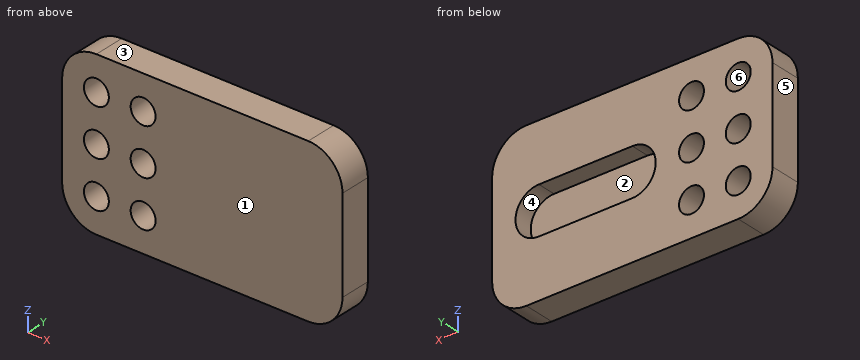
```python
from build123d import *

# Parameters (mm, degrees)
SKETCH1_W           = 180
SKETCH1_H           = 104
BOSS_EXTRUDE1_DEPTH = 20
FILLET1_R           = 22
SKETCH3_R           = 8
CUT_EXTRUDE1_DEPTH  = 20
CUT_EXTRUDE2_DEPTH  = 12


with BuildPart() as part:
    # Sketch1 → Boss-Extrude1 (new body)
    with BuildSketch(Plane(origin=(0, 0, 0), x_dir=(1, 0, 0), z_dir=(0, 1, 0))):
        Rectangle(SKETCH1_W, SKETCH1_H)
    extrude(amount=BOSS_EXTRUDE1_DEPTH)

    # Fillet1
    fillet1_edges = [part.edges().sort_by_distance(p)[0] for p in [
        (90, 10, 52),
        (-90, 10, 52),
        (-90, 10, -52),
        (90, 10, -52),
    ]]
    fillet(fillet1_edges, radius=FILLET1_R)

    # Sketch3 → Cut-Extrude1 (cut)
    with BuildSketch(Plane(origin=(0, 20, 0), x_dir=(1, 0, 0), z_dir=(0, 1, 0))):
        with Locations(Location((-68, 30, 0), (0, 0, 270))):
            Circle(SKETCH3_R)
        with Locations(Location((-68, 0, 0), (0, 0, 270))):
            Circle(SKETCH3_R)
        with Locations(Location((-68, -30, 0), (0, 0, 270))):
            Circle(SKETCH3_R)
        with Locations(Location((-38, -30, 0), (0, 0, 270))):
            Circle(SKETCH3_R)
        with Locations(Location((-38, 0, 0), (0, 0, 270))):
            Circle(SKETCH3_R)
        with Locations(Location((-38, 30, 0), (0, 0, 270))):
            Circle(SKETCH3_R)
    extrude(amount=-CUT_EXTRUDE1_DEPTH, mode=Mode.SUBTRACT)

    # Sketch4 → Cut-Extrude2 (cut)
    with BuildSketch(Plane(origin=(0, 20, 0), x_dir=(1, 0, 0), z_dir=(0, 1, 0))):
        with BuildLine():
            Line((0, 15), (60, 15))
            ThreePointArc((60, 15), (75, 0), (60, -15))
            Line((60, -15), (0, -15))
            ThreePointArc((0, -15), (-15, 0), (0, 15))
        make_face()
    extrude(amount=-CUT_EXTRUDE2_DEPTH, mode=Mode.SUBTRACT)


solid = part.part
```
Geometry: final body of the model. Coordinates: model frame, mm. Face numbers are marked on the shaded views. A direction names the side the tool comes from. Give positions to 0.01 mm unless a question says otherwise; leave off trailing zeros. Write each loop counter-clockwise with the first axis right and the second up, starting at its lowest first coordinate (ties: lowest second). Pieces come first, ordered by that corner, then holes.
1. Section query B-B, the plane y = 10. Return loops of the section in (x, z).
2. Section query D-D, the plane x = 20. Return loops of the section in (y, z).
3. Section query C-C, the plane z = 0. Return loops of the section in (x, y).
4. Draft query along Z for the marked faces 3, 4, 5 and 6. Return one class per face: released by +Z, released by -Z, zero draft, split by the parting line, or undercut.
5. Line query: probe 1 along X at (y, z) = (6.5, -30); probe 2 along Z at (x, y) = (8, 8.5); probe 3 along Z at (x, y) = (-71.5, 14). Output: solid intervals per line, ascending.
6. Pin query (flat end, axial travel): P1, Ø9.5, axis at x = -68, z = -30, coming from the +Y side. Return the tip coordinate at first contact, or that it passes through.
7. Section query A-A, the plane x = -38. Return loops of the section in (y, z), then the cut area to 3 significant figures.
8. Reachability of the marked faces 1 and 2 from +Z, -Z, +X, -X, +Y, -Y: full face, straight path, thin tool, end or side. Return the list, or none.
Computed:
1. outline: (-90, -30) arc R22 ccw to (-68, -52) - (68, -52) arc R22 ccw to (90, -30) - (90, 30) arc R22 ccw to (68, 52) - (-68, 52) arc R22 ccw to (-90, 30) - close; hole circle Ø16 at (-68, -30); hole circle Ø16 at (-68, 0); hole circle Ø16 at (-68, 30); hole circle Ø16 at (-38, -30); hole circle Ø16 at (-38, 0); hole circle Ø16 at (-38, 30); hole (0, -15) - (60, -15) arc R15 ccw to (60, 15) - (0, 15) arc R15 ccw to start
2. outline: (0, -52) - (20, -52) - (20, -15) - (8, -15) - (8, 15) - (20, 15) - (20, 52) - (0, 52) - close
3. outline: (-90, 0) - (-76, 0) - (-76, 20) - (-90, 20) - close; (-60, 0) - (-46, 0) - (-46, 20) - (-60, 20) - close; (-30, 0) - (90, 0) - (90, 20) - (75, 20) - (75, 8) - (-15, 8) - (-15, 20) - (-30, 20) - close
4. face 3: released by +Z
4. face 4: undercut
4. face 5: zero draft
4. face 6: undercut
5. probe 1: x = -90 to -76, -60 to -46, -30 to 90
5. probe 2: z = -52 to -15, 15 to 52
5. probe 3: z = -51.72 to -37.19, -22.81 to -7.19, 7.19 to 22.81, 37.19 to 51.72
6. P1: passes through
7. outline: (0, -52) - (20, -52) - (20, -38) - (0, -38) - close; (0, -22) - (20, -22) - (20, -8) - (0, -8) - close; (0, 8) - (20, 8) - (20, 22) - (0, 22) - close; (0, 38) - (20, 38) - (20, 52) - (0, 52) - close
7. area: 1,120 mm2
8. face 1: +Z, -Z, +X, -X, -Y
8. face 2: +Y
